The model under review builds one solid part; all positions refer to its coordinate system, in mm. Round coordinates to 2 decimals unless told otherwise and drop trailing zeros. Order: outer loops, then holes, each group sorted by start corner. A loop starts at its lowest first (then second) coordinate and runs counter-clockwise, first axis right, second up.
```python
from build123d import *

# Parameters (mm, degrees)
F0_R      = 75.62278
F1_DEPTH  = 75.692
F2_R      = 34.789881
F3_DEPTH  = 148.844
F3_FACE_R = 34.789881
F4_DEPTH  = 287.274


with BuildPart() as f1:
    # F0 (on Top) → F1 (new body)
    with BuildSketch(Plane.XY):
        Circle(F0_R)
    extrude(amount=F1_DEPTH)

    # F2 (on face) → F3 (join)
    with BuildSketch(Plane.XY.offset(75.692)):
        Circle(F2_R)
    extrude(amount=-F3_DEPTH)

    # F3_face (on face) → F4 (cut)
    with BuildSketch(Plane(origin=(0, 0, -73.152), x_dir=(1, 0, 0), z_dir=(0, 0, -1))):
        Circle(F3_FACE_R)
    extrude(amount=-F4_DEPTH, mode=Mode.SUBTRACT)


solid = f1.part
```
(1) To check wall thickness, follow probe 1 along Y at (x, z) = (0, 49); probe 2 along Y at (x, z) = (-14.5, 51.5); probe 3 along X at (y, z) = (3, 32). State the ranges of each line that lie inside material, in increasing order.
Data:
probe 1: y = -75.62 to -34.79, 34.79 to 75.62
probe 2: y = -74.22 to -31.62, 31.62 to 74.22
probe 3: x = -75.56 to -34.66, 34.66 to 75.56
(2) Draft analysis for pull direction X (two halves, no side actions). For faces 1 (the flat face through (33, -16, 0)), 2 (the cylindrical face through (-4.529, -34.494, 37.316)), 3 (the cylindrical face through (-9.84, 74.98, 37.32)), state which applies: pulls with the +X half, pulls with the -X half, needs draft (parallel to the pull), parting line crosses it, or undercut.
Data:
face 1: needs draft
face 2: undercut
face 3: parting line crosses it
(3) Consider section D-D (x = 48). Write out the cut boundary in (y, z).
Data:
outline: (-58.44, 0) - (58.44, 0) - (58.44, 75.69) - (-58.44, 75.69) - close
(4) Consider section C-C (z = 63). Write out the cut boundary in (x, y), and give its area (3 significant figures).
Data:
outline: circle Ø151.25 at (0, 0); hole circle Ø69.58 at (0, 0)
area: 14,200 mm2
(5) Insertion check: pin 1 (10 mm diameter, centred on y = -2.5, z = 39.5, fed in from +X); pin 2 (1.5 mm diameter, centred on x = 14.5, z = 12.5, fed in from +Y); pin 3 (4 mm diameter, centred on x = 26, z = 49.5, fed in from -Y); pin 4 (6 mm diameter, centred on y = 10.5, z = 28, fed in from -X). Each pin has a flat end and moves straight along its axis. Give the tip position at first contact, or say it passes through.
Data:
pin 1: stops at x = 75.62
pin 2: stops at y = 74.36
pin 3: stops at y = -71.71
pin 4: stops at x = -75.25
(6) Consider section A-A (x = 0). Write out the cut boundary in (y, z), and give its area (3 significant figures).
Data:
outline: (-75.62, 0) - (-34.79, 0) - (-34.79, 75.69) - (-75.62, 75.69) - close; (34.79, 0) - (75.62, 0) - (75.62, 75.69) - (34.79, 75.69) - close
area: 6,180 mm2
